Part print with two shaded views. Sizes in mm from the minimum x, y, z corner. Round coordinates to 2 decimals unless told otherwise and drop trailing zeros. Loops run counter-clockwise (first coordinate to the right, second up) from the corner with the lowest first, then second, coordinate; pieces in that order, holes last. Notation, with made-up numbers: M 57,-14.5 L 82,-14.5 A21 cw 82,1.5 Z; hole C -21.75,70.25 d8. An arc over 180 degrees is marked long. Use a Markdown table: item, result. Add a question column.
Item 1: Pin check, flat tips, straight feed: P1, Ø1.5, axis at x = 152, y = 1.5, coming from the -Z side; P2, Ø1.5, axis at y = 2, z = 9, coming from the +X side. Stop position of each tip, or through.
Item 2: Saw through at B-B on z = 26.5. Write the cut outline in (x, y), then the cut area to 3 significant figures.
Item 3: Saw through at C-C on y = 1.1. Write the cut outline in (x, z), then the cut area to 3 significant figures.
Item 4: Saw through at D-D on x = 56.5. Write the cut outline in (y, z).
Item 5: Saw through at A-A on x = 93.41. Write the cut outline in (y, z), then the cut area to 3 significant figures.
Item 6: Wall check: L1, parallel to Z at x = 143, y = 0.7; L2, parallel to X at y = 0.2, z = 81.5; L3, parallel to X at y = 0.4, z = 21. Give the ranges that are in metal, low to high. Write a range as from..to.
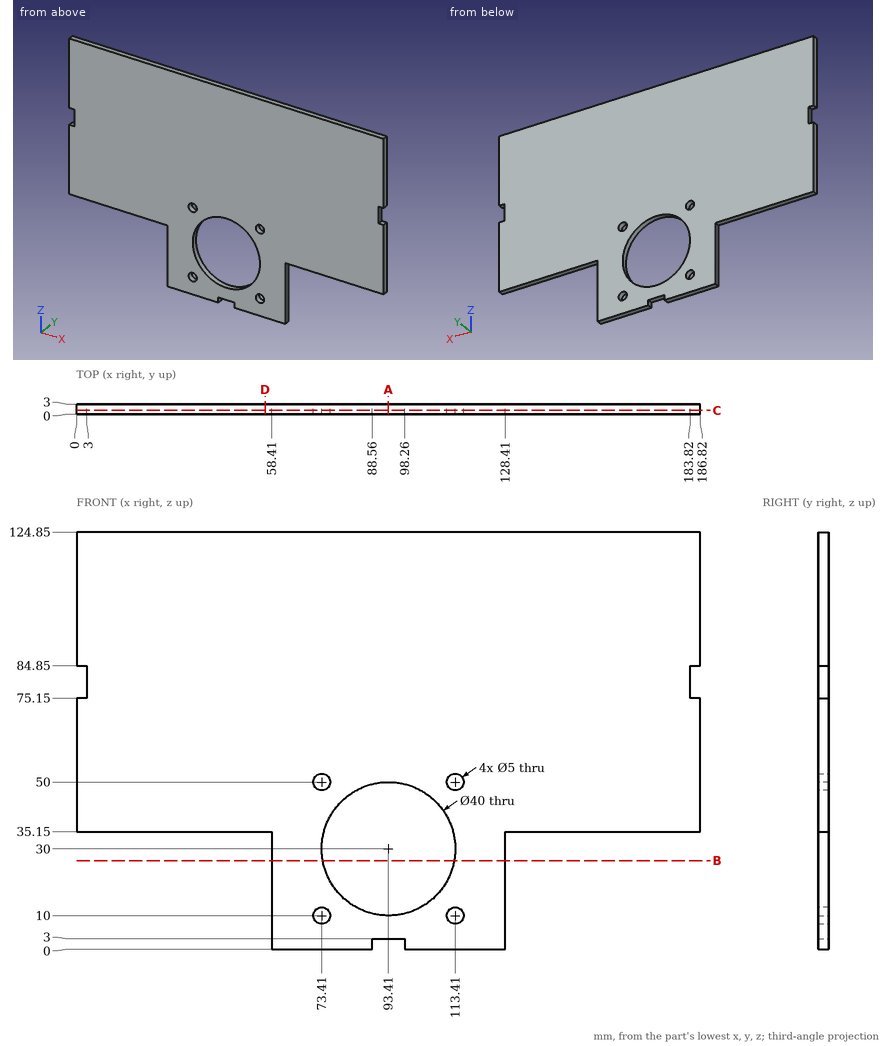
Entries:
| question | item | result |
|---|---|---|
| 1 | P1 | z = 35.15 |
| 1 | P2 | x = 128.41 |
| 2 | outline | M 58.41,0 L 73.72,0 L 73.72,3 L 58.41,3 Z; M 113.1,0 L 128.41,0 L 128.41,3 L 113.1,3 Z |
| 2 | area | 91.9 mm2 |
| 3 | outline | M 0,35.15 L 58.41,35.15 L 58.41,0 L 88.56,0 L 88.56,3 L 98.26,3 L 98.26,0 L 128.41,0 L 128.41,35.15 L 186.82,35.15 L 186.82,75.15 L 183.82,75.15 L 183.82,84.85 L 186.82,84.85 L 186.82,124.85 L 0,124.85 L 0,84.85 L 3,84.85 L 3,75.15 L 0,75.15 Z; hole C 73.41,10 d5; hole C 73.41,50 d5; hole C 93.41,30 d40; hole C 113.41,10 d5; hole C 113.41,50 d5 |
| 3 | area | 17,800 mm2 |
| 4 | outline | M 0,35.15 L 3,35.15 L 3,124.85 L 0,124.85 Z |
| 5 | outline | M 0,3 L 3,3 L 3,10 L 0,10 Z; M 0,50 L 3,50 L 3,124.85 L 0,124.85 Z |
| 5 | area | 246 mm2 |
| 6 | L1 | 35.15..124.85 |
| 6 | L2 | 3..183.82 |
| 6 | L3 | 58.41..75.55, 111.27..128.41 |
